Print and shaded views of the part. All mm, measured from the part's lowest x, y and z. Give positions to 0.01 mm unless a question says otherwise; leave off trailing zeros. Loops run counter-clockwise (first coordinate to the right, second up) from the corner with the lowest first, then second, coordinate; pieces in that order, holes last.
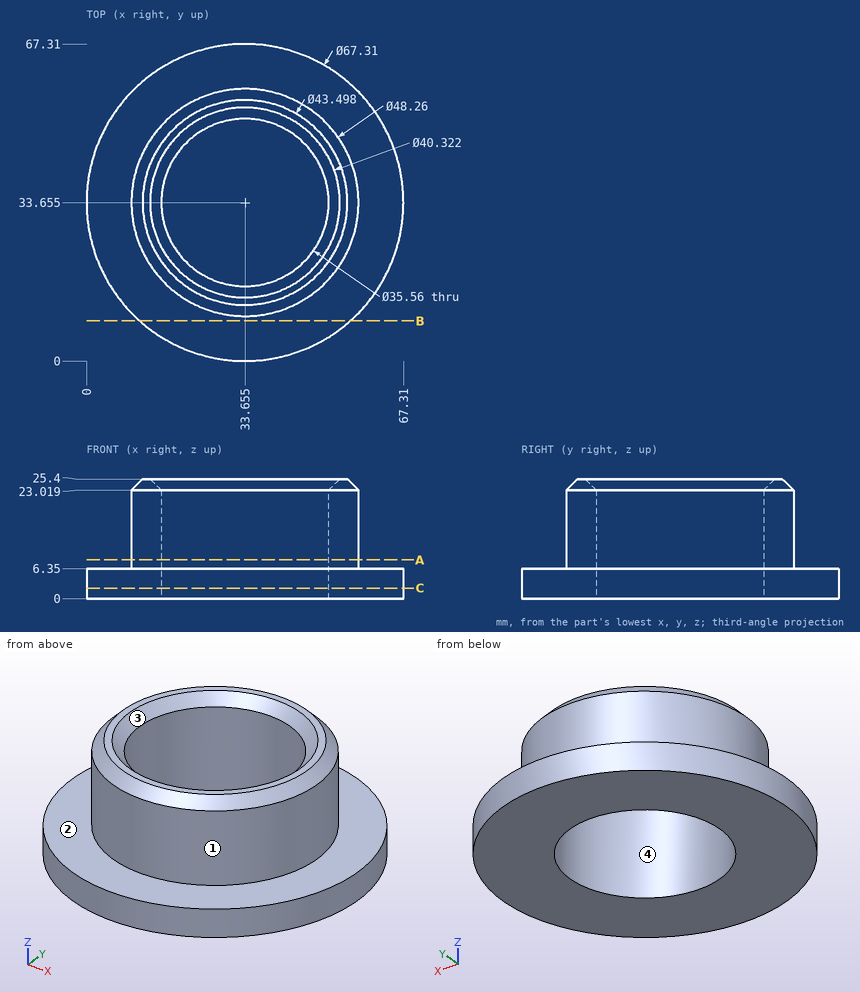
1. Drop flat-ended pins along their axis: pin 1 (10 mm diameter, centred on x = 43, z = 20, fed in from -Y); pin 2 (12 mm diameter, centred on x = 15, z = 15.5, fed in from -Y); pin 3 (12 mm diameter, centred on y = 48, z = 22, fed in from -X) (1 decimal). Give the stop position or say it passes through.
Responses:
pin 1: stops at y = 9.92
pin 2: stops at y = 13.11
pin 3: stops at x = 11
2. Pull direction X, two halves, no side cores. Call the marked faces 1, 2, 3 and 4: released by +X, released by -X, zero draft, split by the parting line, or undercut.
Responses:
face 1: split by the parting line
face 2: zero draft
face 3: undercut
face 4: undercut
3. Saw through at B-B, the plane y = 8.5. List the corners of the cut face in (x, z), and give its area (3 significant figures).
Responses:
outline: (11.3, 0) - (56.01, 0) - (56.01, 6.35) - (11.3, 6.35) - close
area: 284 mm2
4. Probe line 1 along X through (y, z) = (34, 21); line 2 along X through (y, z) = (23.5, 23.75) (1 decimal); line 3 along Z through (x, y) = (6, 35.5). List the from-to ranges inside material, lowest first.
Responses:
line 1: x = 9.53 to 15.88, 51.43 to 57.78
line 2: x = 12.6 to 18.2, 49.1 to 54.7
line 3: z = 0 to 6.35
5. Saw through at A-A, the plane z = 8.25. List the corners of the cut face in (x, y) (1 decimal), and give its area (3 significant figures).
Responses:
outline: circle Ø48.3 at (33.7, 33.7); hole circle Ø35.6 at (33.7, 33.7)
area: 836 mm2
6. Saw through at C-C, the plane z = 2.25. List the corners of the cut face in (x, y) (1 decimal).
Responses:
outline: circle Ø67.3 at (33.7, 33.7); hole circle Ø35.6 at (33.7, 33.7)
